Drawing for the job (mm, zero at the part's lowest x, y, z). Give positions to 0.01 mm unless a question says otherwise; leave off trailing zeros. Write each loop counter-clockwise with the first axis right and the second up, starting at its lowest first coordinate (ties: lowest second). Pieces come first, ordered by that corner, then holes. Notation, with made-up numbers: (46, 36) - (97, 36) arc R8 cw to (97, 49) - close; hole circle Ø11 at (49, 64.25). An arc over 180 degrees is marked (long way). Write item = value, one per line. Start each with the question number.
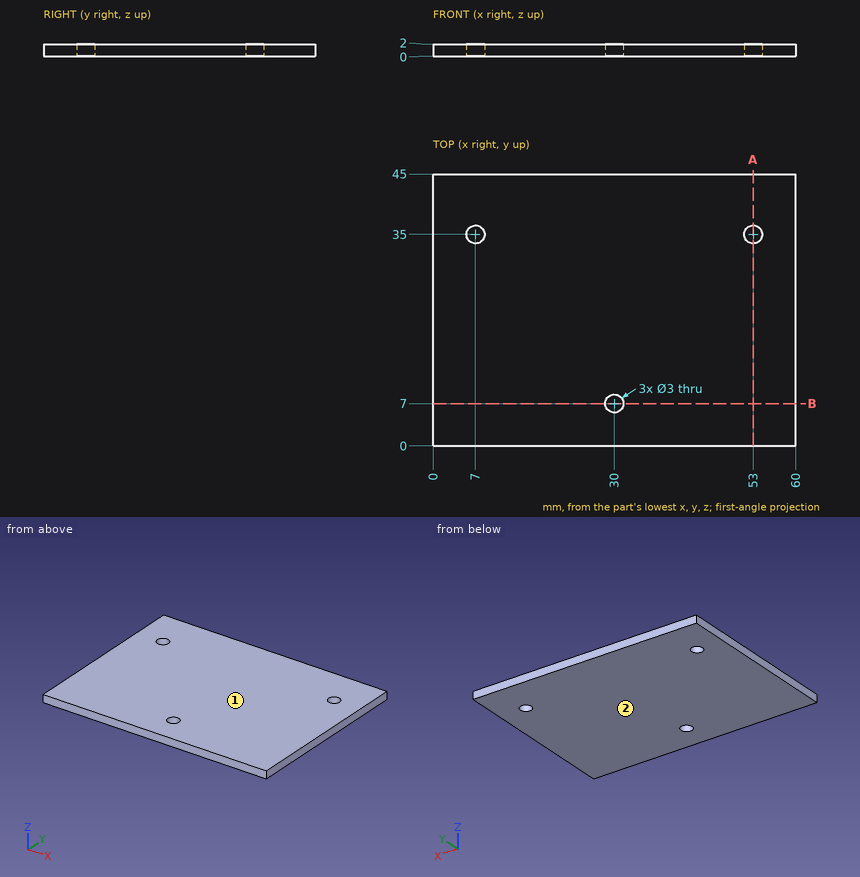
1. Cut at B-B (y = 7). Give the cut face in (x, z).
2. Wall check: line 1 along Y through (x, z) = (7, 1.45); line 2 along Y through (x, z) = (30, 0.7). Give the ranges that are in metal, low to high.
3. Cut at A-A (x = 53). Give the cut face in (y, z), then the cut area to 3 significant figures.
4. Pin check, flat tip, straight feed: pin 1 Ø4 at (x, y) = (30, 7) entering from -Z. Stop position of the tip, or through.
5. Mould opens along Z. For the marked faces 1 and 2 say: +Z half, -Z half, draft (parallel to the pull), parting line (faces both ways), or undercut.
Output:
q1.outline = (0, 0) - (28.5, 0) - (28.5, 2) - (0, 2) - close; (31.5, 0) - (60, 0) - (60, 2) - (31.5, 2) - close
q2.line_1 = 0 to 33.5, 36.5 to 45
q2.line_2 = 0 to 5.5, 8.5 to 45
q3.outline = (0, 0) - (33.5, 0) - (33.5, 2) - (0, 2) - close; (36.5, 0) - (45, 0) - (45, 2) - (36.5, 2) - close
q3.area = 84.0 mm2
q4.pin_1 = 0
q5.face_1 = +Z half
q5.face_2 = -Z half
